Read the model definition and answer for the solid it produces. Units are mm, in the model's axes. A direction names the side the tool comes from. Round coordinates to 2 decimals unless told otherwise and drop trailing zeros. Order: outer loops, then holes, each group sorted by start corner. A loop starts at its lowest first (then second) coordinate and runs counter-clockwise, first axis right, second up. Notation, with made-up numbers: (35.25, -11.75) - (85.25, -11.75) arc R18 cw to (85.25, 23.25) - close; hole circle Ø7 at (-4, 25.25). An arc over 180 degrees is marked (long way). Answer as a JSON object with one key per item and string values. Group by question number.
Q1. A cutting plane is placed at B-B on y = 10.5. Determine the outline of the cut face in (x, z), and give its area (3 significant figures).
Q2. Consider line 1 (X direction, y = 7.5, z = 23.5); line 2 (X direction, y = 32, z = 7); line 3 (Z direction, x = 13, y = 5.5). Determine where each line is inside the solid, lowest interval first.
Q3. Given pin 1 Ø8 at (x, y) = (-14.5, 15) entering from +Z; pin 2 Ø3 at (y, z) = (22.5, 22) entering from +X; pin 3 Ø5 at (y, z) = (10.5, 13) entering from +X, each flat-ended and moving along its own axis, determine where each tip first touches the part or whether it passes through.
Q4. A cutting plane is placed at C-C on x = 0. Determine the outline of the cut face in (y, z).
Q5. The mould has two halves that part along X. Classify faces 1 (the cylindrical face through (1, 22.18, 45.49)), 2 (the cylindrical face through (0.85, 22.18, 38.49)), 3 (the flat face through (-42, 22, 0)): pulls with the +X half, pulls with the -X half, needs draft (parallel to the pull), parting line crosses it, or undercut.
Q6. A cutting plane is placed at A-A on z = 7.5. Determine the outline of the cut face in (x, y), and give its area (3 significant figures).
Q7. A tool of negligible diameter and unlimited length cuts with its end or side. For faces 4 (the flat face through (6.95, 45, 38.02)), 5 (the cylindrical face through (41.4, 19.15, 6.99)), from which of +Z, -Z, +X, -X, +Y, -Y can it reach the whole face along a straight path? Write none if from no direction.
Q8. A cutting plane is placed at D-D on z = 26. Determine the outline of the cut face in (x, y).
Autodesk Inventor part; units mm, degrees
ref_plane "YZ Plane" through (0, 0, 0) normal (1, 0, 0) x (0, 1, 0)
ref_plane "XZ Plane" through (0, 0, 0) normal (0, 1, 0) x (-1, 0, 0)
ref_plane "XY Plane" through (0, 0, 0) normal (0, 0, 1) x (1, 0, 0)
sketch "Sketch1" plane through (0, 0, 0) normal (0, 1, 0) x (-1, 0, 0)
  circle A0 centre (0, 0) radius 45.5
  circle A1 centre (0, 0) radius 38.5
  line L0 (-45.5, 0) -> (-38.5, 0)
  line L1 (38.5, 0) -> (45.5, 0)
  dimension "d1" = 7
  dimension "d4" = 91
extrude "Extrusion1" add sketch "Sketch1" along normal blind 45 contours L1 A1 L0 A0 picked at (-42.8352, 3.1533)
ref_plane "Work Plane1" through (45.5, 0, 0) normal (1, 0, 0) x (0, 1, 0)
sketch "Sketch2" plane through (45.5, 0, 0) normal (1, 0, 0) x (0, 1, 0)
  arc A0 (22, 0) -> (12, 10) centre (12, 0) ccw
  line L0 (0, 0) -> (0, 45.5)
  line L1 (0, 0) -> (45, 0)
  line L2 (22, 0) -> (22, 0)
  line L3 (0, 0) -> (45, 0)
  line L4 (2, 0) -> (2, 0)
  line L5 (22, 0) -> (2, 0)
  line L6 (12, 10) -> (0, 10)
  line L7 (0, 38.5) -> (0, 0)
  line L8 (0, 10) -> (0, 0)
  line L9 (0, 0) -> (12, 0)
  dimension "d7" = 20
  dimension "KisFogaskerekBesulyesztese" = 12
  dimension "d9" = 0
extrude "Extrusion2" cut sketch "Sketch2" against normal blind 50
equation "\"d1\" = PVCfalVastagsag"
equation "\"d4\" = KulsoAtmeroPVCcso"
equation "\"KisFogaskerekBesulyesztese\" = KisFogaskerekBesulyesztes"
properties part number "BurkolatPVCszenzorFedel" material "PVC-Piping"
Result set:
{
 "1": {"outline": "(-45.5, 0) - (-38.5, 0) arc R38.5 cw to (37.18, 10) - (44.39, 10) arc R45.5 ccw to start", "area": "853 mm²"},
 "2": {"line 1": "x = -38.96 to -30.5, 30.5 to 38.96", "line 2": "x = -44.96 to -37.86, 37.86 to 44.96", "line 3": "z = 36.24 to 43.6"},
 "3": {"pin 1": "stops at z = 44.27", "pin 2": "stops at x = 40.62", "pin 3": "stops at x = 44.27"},
 "4": {"outline": "(0, 38.5) - (45, 38.5) - (45, 45.5) - (0, 45.5) - close"},
 "5": {"face 1": "parting line crosses it", "face 2": "undercut", "face 3": "needs draft"},
 "6": {"outline": "(-44.88, 0) - (-37.76, 0) - (-37.76, 45) - (-44.88, 45) - close; (37.76, 18.61) - (44.88, 18.61) - (44.88, 45) - (37.76, 45) - close", "area": "508 mm²"},
 "7": {"face 4": "+Z, -Z, +X, -X, +Y", "face 5": "-Z, +X, -Y"},
 "8": {"outline": "(-37.34, 0) - (-28.39, 0) - (-28.39, 45) - (-37.34, 45) - close; (28.39, 0) - (37.34, 0) - (37.34, 45) - (28.39, 45) - close"}
}
